For this review, take the finished solid that the model builds, in its own axes (mm). A direction names the side the tool comes from. Round coordinates to 2 decimals unless told otherwise and drop trailing zeros. Order: outer loops, then holes, each group sorted by start corner. A loop starts at its lowest first (then second) coordinate and runs counter-clockwise, first axis right, second up. Notation, with made-up numbers: (28.5, 58) - (79.5, 58) arc R21 ccw to (79.5, 76) - close; hole circle Ø8 at (22, -1.75). An arc over 180 degrees is marked (long way). Write each question's results on one line, items separated by ' | '. Start each with the question number.
(1) For L1, parallel to Z at x = 26, y = 23; L2, parallel to X at y = -9, z = 19.5; L3, parallel to Y at x = -2, z = 10.5, list the stretches that pass through material, from the lowest coordinate up. Write a range as from..to.
(2) Take a section at B-B, the plane z = 17.5. Give the number of separate pieces and of enclosed holes in the cut face, plus the area to 3 significant figures.
(3) Take a section at A-A, the plane y = -8. Give the boundary of the cut face in (x, z), plus the area to 3 significant figures.
(4) Insertion check: pin 1 Ø10 at (x, z) = (-11, 11) entering from +Y; pin 2 Ø9.5 at (x, z) = (-13.21, 17.5) entering from -Y; pin 3 Ø18.5 at (x, z) = (-4, 14.5) entering from -Y. Each pin has a flat end and moves straight along its axis. Give the tip position at first contact, or say it passes through.
(5) For faces 1 (the flat face through (0, -24, 17)), 2 (the cylindrical face through (4.642, -47.918, 34.715)), 3 (the flat face through (26, -68, 14)), 4 (the cylindrical face through (-12.56, 4.49, 14.57)), 5 (the flat face through (14, 16, 33)), list the 3-axis set-ups (+Z, -Z, +X, -X, +Y, -Y) from which the entire face can be reached by the end or side of a thin tool; tool diameter is ignored.
(6) Draft analysis for pull direction X (two halves, no side actions). For faces 6 (the flat face through (28, 26, 17)), 7 (the flat face through (2, 5.473, 17)), 8 (the flat face through (26, -27, 17)), state which applies: pulls with the +X half, pulls with the -X half, needs draft (parallel to the pull), parting line crosses it, or undercut.
```python
from build123d import *

# Parameters (mm, degrees)
F1_DEPTH    = 35
F3_T        = 2
F3_T3_DEPTH = 39
F4_R        = 3
F5_DEPTH    = 25
F6_R        = 3
F7_DEPTH    = 5.9
F8_R        = 0.99999
F9_R        = 3
F10_DEPTH   = 25
F11_R       = 3
F12_DEPTH   = 25


# Not quite as in the source:
# - a fillet or chamfer is up to 0.001 mm smaller than in the source, because OpenCascade refuses the exact size
# - a shell that OpenCascade refuses in one call is made with other operations: the cavity is built on its own and cut out
# - a feature names something its author has since deleted; it is built from what else it names


with BuildPart() as f1:
    # F0 (on Top) → F1 (new body)
    with BuildSketch(Plane.XY):
        Polygon((0, -35.5268927627), (-25, -35.5268927627), (26, -61.7087109445), (26, -75.1632548192), (30, -75.1632548192), (30, 43.5640147483), (30, 46.7083996511), (26, 43.5640147483), (-25, 3.4731072373), (0, 3.4731072373), (0, -11.5268927627), (-25, -11.5268927627), (-25, -13.5268927627), (0, -13.5268927627), align=None)
        Polygon((3, -38.5268927627), (3, 3.4731072373), (26, 3.4731072373), (26, -58.7087109445), (-12.7289108932, -38.5268927627), align=None, mode=Mode.SUBTRACT)
    extrude(amount=F1_DEPTH)

    # F3: shell of thickness 2, made by hand


with BuildPart() as f3_core1:
    # F3_t2: copy of F1
    add(f1.part)

    # the walls: a layer under each face that stays
    f3_faces = [f3_core1.faces().sort_by_distance(p)[0] for p in [
        (-12.5, 3.4731072373, 17.5),
        (2.5, -14.227427584, 35),
        (-4.8644554466, -38.5268927627, 17.5),
        (6.6355445534, -48.6178018536, 17.5),
        (26, -27.6178018536, 17.5),
        (14.5, 3.4731072373, 17.5),
        (3, -17.5268927627, 17.5),
        (30, -14.227427584, 17.5),
        (28, -75.1632548192, 17.5),
        (26, -68.4359828818, 17.5),
        (0.5, -48.6178018536, 17.5),
        (-12.5, -35.5268927627, 17.5),
        (0, -24.5268927627, 17.5),
        (-12.5, -13.5268927627, 17.5),
        (-25, -12.5268927627, 17.5),
        (-12.5, -11.5268927627, 17.5),
        (2.5, -14.227427584, 0),
        (0, -4.0268927627, 17.5),
    ]]
    thicken(f3_faces, amount=-F3_T, mode=Mode.SUBTRACT)

    # F3_s4 → F3_t3 (cut)
    with BuildSketch(Plane.XY.offset(-2)):
        Polygon((-0.02, 3.4531072373), (0, 5.4731072373), (2, 5.4731072373), (2, 3.4731072373), align=None)
        Polygon((-12.7196684188, -38.5291564534), (-12.7289108932, -36.5268927627), (-20.8947564215, -36.5268927627), (-13.6531583366, -40.3005236892), align=None)
        Polygon((25.9892424744, -58.6909746353), (25.0757525566, -60.482341871), (28, -62.0061810098), (28, -58.7087109445), align=None)
        Polygon((25.98, 3.4531072373), (28, 3.4731072373), (28, 5.4731072373), (26, 5.4731072373), align=None)
        Polygon((3.02, 3.4531072373), (3, 5.4731072373), (1, 5.4731072373), (1, 3.4731072373), align=None)
        Polygon((25.9708659413, -61.7265033297), (28, -61.7087109445), (28, -60.4872961474), (26.9134058716, -59.9294724238), align=None)
        Polygon((-0.02, -35.5068927627), (0, -37.5268927627), (2, -37.5268927627), (2, -35.5268927627), align=None)
        Polygon((-0.02, -13.5468927627), (2, -13.5268927627), (2, -11.5268927627), (0, -11.5268927627), align=None)
        Polygon((-0.02, -11.5068927627), (0, -13.5268927627), (2, -13.5268927627), (2, -11.5268927627), align=None)
    extrude(amount=F3_T3_DEPTH, mode=Mode.SUBTRACT)


with BuildPart() as f1_1:
    add(f1.part)

    # what is left inside the walls is the cavity
    f3_cavity = [f3_core1.part.solids().sort_by_distance(p)[0] for p in [
        (2.784469, 25.288934, 22.666667),
    ]]
    add(f3_cavity, mode=Mode.SUBTRACT)

    # F4 (on face) → F5 (cut)
    with BuildSketch(Plane(origin=(28, 0, 0), x_dir=(0, -1, 0), z_dir=(-1, 0, 0))):
        with Locations((-16.8671440333, 17.5)):
            Circle(F4_R)
    extrude(amount=-F5_DEPTH, mode=Mode.SUBTRACT)

    # F6 (on face) → F7 (cut)
    with BuildSketch(Plane(origin=(0, 5.4731072373, 0), x_dir=(-1, 0, 0), z_dir=(0, 1, 0))):
        with Locations((13.21292707, 17.5)):
            Circle(F6_R)
    extrude(amount=-F7_DEPTH, mode=Mode.SUBTRACT)

    # F8 (radius 1 in the source; OpenCascade refuses exactly that, so slightly less here)
    f8_edges = [f1_1.edges().sort_by_distance(p)[0] for p in [
        (2.5, 25.090753, 35),
        (2.5, 25.090753, 0),
        (-25, 3.473107, 17.5),
        (-12.5, 3.473107, 35),
        (-12.5, 3.473107, 0),
        (0, 3.473107, 17.5),
        (0, -11.526893, 17.5),
        (0, -13.526893, 17.5),
        (-25, -13.526893, 17.5),
        (-12.5, -13.526893, 0),
        (-12.5, -13.526893, 35),
        (-25, -11.526893, 17.5),
        (0, -35.526893, 17.5),
        (-25, -35.526893, 17.5),
        (0.5, -48.617802, 35),
        (0.5, -48.617802, 0),
        (26, -61.708711, 17.5),
        (3, -17.526893, 35),
        (6.635545, -48.617802, 35),
        (26, -27.617802, 35),
        (14.5, 3.473107, 35),
        (3, -17.526893, 0),
        (14.5, 3.473107, 0),
        (26, -27.617802, 0),
        (6.635545, -48.617802, 0),
        (26, -75.163255, 17.5),
        (3, -38.526893, 17.5),
        (26, -58.708711, 17.5),
        (26, 3.473107, 17.5),
        (2.772109, 25.304657, 33),
        (2.772109, 25.304657, 2),
        (0, -4.026893, 0),
        (-12.5, -11.526893, 0),
        (0, -24.526893, 0),
        (-12.5, -35.526893, 0),
        (26, -68.435983, 0),
        (0, -4.026893, 35),
        (-12.5, -11.526893, 35),
        (0, -24.526893, 35),
        (-12.5, -35.526893, 35),
        (26, -68.435983, 35),
        (30, -75.163255, 17.5),
        (28, 5.473107, 17.5),
    ]]
    fillet(f8_edges, radius=F8_R)

    # F9 (on face) → F10 (cut)
    with BuildSketch(Plane(origin=(26, 0, 0), x_dir=(0, -1, 0), z_dir=(-1, 0, 0))):
        with Locations((50.3810942173, 17.5)):
            Circle(F9_R)
        with Locations((41.8810732663, 17.5000000745)):
            Circle(F9_R)
    extrude(amount=-F10_DEPTH, mode=Mode.SUBTRACT)

    # F11 (on face) → F12 (cut)
    with BuildSketch(Plane(origin=(26, 0, 0), x_dir=(0, -1, 0), z_dir=(-1, 0, 0))):
        with Locations((67.9058432579, 17.5)):
            Circle(F11_R)
    extrude(amount=-F12_DEPTH, mode=Mode.SUBTRACT)


solid = f1_1.part
```
Results below:
1) L1: z = 0..2, 33..35 | L2: x = 0..3, 26..30 | L3: y = -47.33..-44.12, -38.53..-35.53, -13.53..-11.53, 3.47..5.47
2) separate pieces: 5 | enclosed holes: 0 | area: 778 mm^2
3) outline: (0, 1) arc R1 ccw to (1, 0) - (2, 0) arc R1 ccw to (3, 1) - (3, 34) arc R1 ccw to (2, 35) - (1, 35) arc R1 ccw to (0, 34) - close; (26, 1) arc R1 ccw to (27, 0) - (30, 0) - (30, 35) - (27, 35) arc R1 ccw to (26, 34) - close | area: 244 mm^2
4) pin 1: stops at y = 5.47 | pin 2: stops at y = -44.02 | pin 3: stops at y = -51.06
5) face 1: +Z, -Z, -X | face 2: +Z | face 3: +Z, -Z, -X, -Y | face 4: +Y | face 5: -X, +Y
6) face 6: pulls with the -X half | face 7: needs draft | face 8: undercut
